from build123d import *

# Parameters (mm, degrees)
F3_DEPTH = 215
F4_SIZE  = 79.99999
F5_R     = 6
F6_DEPTH = 50
F7_W     = 116
F7_H     = 90
F8_DEPTH = 5
F9_R     = 10


# Not quite as in the source:
# - a fillet or chamfer is up to 0.001 mm smaller than in the source, because OpenCascade refuses the exact size


with BuildPart() as f3:
    # F2 (on Right) → F3 (new body, symmetric)
    with BuildSketch(Plane.YZ):
        Polygon((-40, 75), (-40, -75), (40, -75), (40, 15), (0, 15), (0, 75), align=None)
    extrude(amount=F3_DEPTH, both=True)

    # F4 (size 80 in the source; OpenCascade refuses exactly that, so slightly less here)
    f4_edges = [f3.edges().sort_by_distance(p)[0] for p in [
        (215, 40, -30),
        (-215, -40, 0),
    ]]
    chamfer(f4_edges, length=F4_SIZE)

    # F5 (on face) → F6 (cut)
    with BuildSketch(Plane(origin=(0, 40, 0), x_dir=(-1, 0, 0), z_dir=(0, 1, 0))):
        with Locations((-105, -45)):
            Circle(F5_R)
        with Locations((-85, -5)):
            Circle(F5_R)
        with Locations((165, -5)):
            Circle(F5_R)
        with Locations((185, -45)):
            Circle(F5_R)
    extrude(amount=-F6_DEPTH, mode=Mode.SUBTRACT)

    # F7 (on face) → F8 (cut)
    with BuildSketch(Plane(origin=(0, 40, 0), x_dir=(-1, 0, 0), z_dir=(0, 1, 0))):
        with Locations((-117, -30)):
            Rectangle(F7_W, F7_H)
        with Locations((197, -30)):
            Rectangle(F7_W, F7_H)
    extrude(amount=-F8_DEPTH, mode=Mode.SUBTRACT)

    # F9
    f9_edges = [f3.edges().sort_by_distance(p)[0] for p in [
        (39.999995, -40, 75),
    ]]
    fillet(f9_edges, radius=F9_R)


solid = f3.part
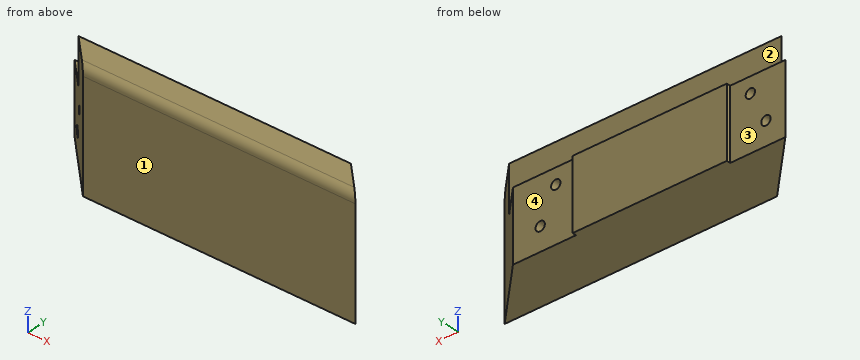
The listing builds one solid part. Answer for the finished solid, in the listing's coordinates (mm). Face numbers are marked on the shaded views. A direction names the side the tool comes from. Coordinates: 2 decimals unless noted, no trailing zeros. Write each loop counter-clockwise with the first axis right and the second up, starting at its lowest first coordinate (ties: lowest second). Pieces come first, ordered by that corner, then holes. Notation, with made-up numbers: (-14, 39.5) - (36, 39.5) arc R24 ccw to (36, 58.5) - close; hole circle Ø5 at (43, 23.25). An arc over 180 degrees is marked (long way). Put each result on its own line as item: value.
1. Find the intervals of material crossed by line 1 along Z through (x, y) = (-165, 11); line 2 along Y through (x, z) = (55, 36); line 3 along X through (y, z) = (-3.5, -7), in increasing order. Write a range as from..to.
Answer sheet:
line 1: z = -75..-11, 1..15
line 2: y = -40..0
line 3: x = -171.5..-170.66, -159.34..79.34, 90.66..178.5
2. A tool of negligible diameter and unlimited length cuts with its end or side. For the marked faces 1, 2, 3 and 4, from which of +Z, -Z, +X, -X, +Y, -Y can it reach the whole face along a straight path? Write none if from no direction.
Answer sheet:
face 1: +Z, -Z, +X, -X, -Y
face 2: +Z, +X, -X, +Y
face 3: +Z, -Z, -X, +Y
face 4: +Z, -Z, +X, +Y
3. The part is cut by section D-D on y = 28. Give the vertices of the cut face in (x, z).
Answer sheet:
outline: (-203, -75) - (147, -75) - (147, 15) - (-203, 15) - close; hole circle Ø12 at (-185, -45); hole circle Ø12 at (-165, -5); hole circle Ø12 at (85, -5); hole circle Ø12 at (105, -45)
4. Flat-ended cylindrical pins translate along their axes: pin 1 Ø6 at (y, z) = (-4.5, 57.5) entering from -X; pin 2 Ø3 at (x, z) = (-163.5, -4) entering from +Y; pin 3 Ø1 at (y, z) = (23, -6) entering from +X. Find the tip coordinate at first contact, or state that the pin passes through.
Answer sheet:
pin 1: stops at x = -173.5
pin 2: stops at y = -10
pin 3: stops at x = 152.5
5. The part is cut by section B-B on x = -185. Give the vertices of the cut face in (y, z).
Answer sheet:
outline: (10, -75) - (35, -75) - (35, -51) - (10, -51) - close; (10, -39) - (35, -39) - (35, 15) - (10, 15) - close
6. The part is cut by section C-C on x = -97.5. Give the vertices of the cut face in (y, z), plus the area to 3 significant figures.
Answer sheet:
outline: (-40, -75) - (40, -75) - (40, 15) - (0, 15) - (0, 75) - (-30, 75) arc R10 ccw to (-40, 65) - close
area: 9,580 mm^2
